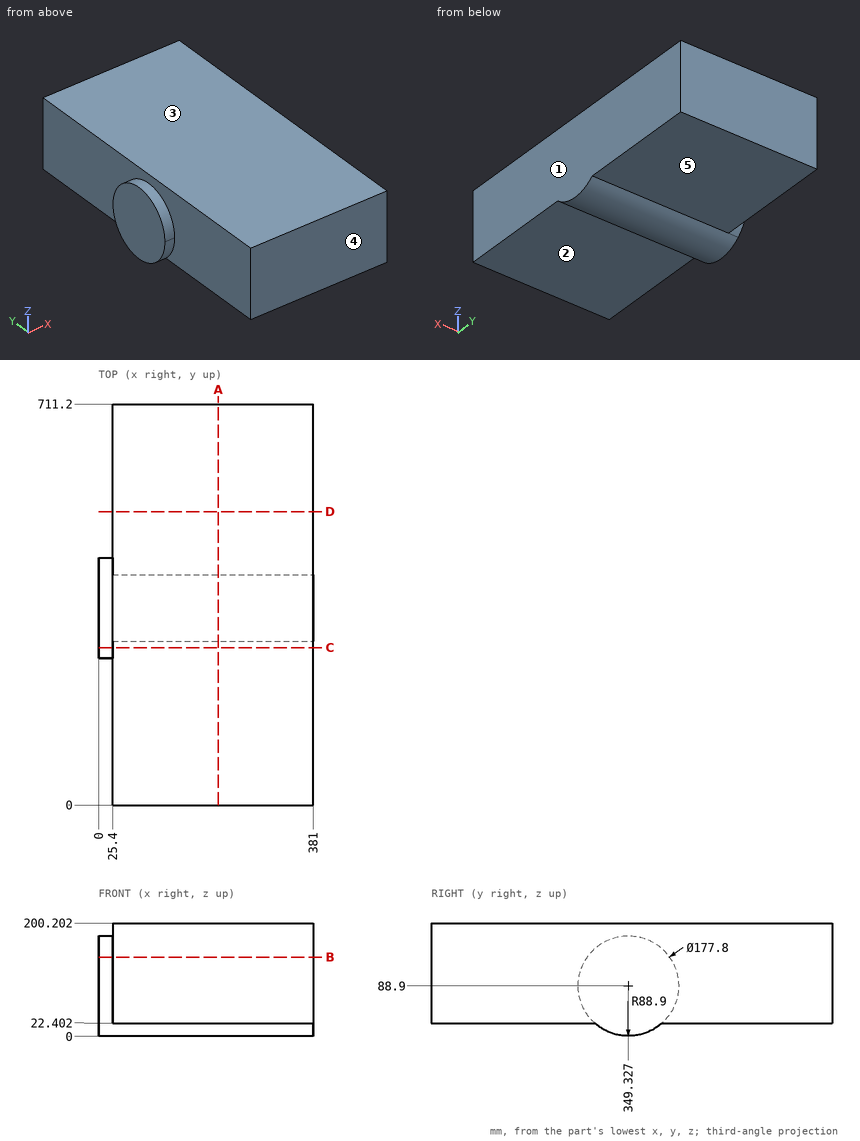
Input: dimensioned drawing with shaded views. Units: mm. Origin: part minimum x, y, z. A direction names the side the tool comes from. Coordinates: 2 decimals unless noted, no trailing zeros. Loops run counter-clockwise (first coordinate to the right, second up) from the corner with the lowest first, then second, coordinate; pieces in that order, holes last. Notation, with made-up numbers: (-7.75, 81) -> (44.25, 81) arc R23 ccw to (44.25, 96) -> close; hole circle Ø2 at (50, 80.5). An arc over 180 degrees is marked (long way). One line per item, written item: value. Start each with the question number.
Q1. Section query C-C, the plane y = 279. Return the cut outline in (x, z).
Q2. Mould query, pull axis Z, two halves, no side actions, for the marked faces 1, 2 and 3. Classes: pulls with the +Z half, pulls with the -Z half, needs draft (parallel to the pull), parting line crosses it, or undercut.
Q3. Contact query for flat-ended pins moving along their axis: P1, Ø1.5, axis at x = 52, y = 216, coming from the -Z side; P2, Ø1, axis at y = 474, z = 24, coming from the -X side. Output: stop coordinate, or through.
Q4. Section query B-B, the plane z = 140. Return the cut outline in (x, y).
Q5. Line query: line 1 along X through (y, z) = (533, 95); line 2 along Z through (x, y) = (41.5, 122); line 3 along Y through (x, z) = (108, 20). Output: solid intervals per line, ascending.
Q6. Section query A-A, the plane x = 212.5. Return the cut outline in (y, z).
Q7. Section query D-D, the plane y = 520.5. Return the cut outline in (x, z), and give its area (3 significant figures).
Q8. Set-up query: the marked faces 4 and 5. Return all of +Z, -Z, +X, -X, +Y, -Y with unobstructed straight access to the full face (end or side cutting, diameter ignored); none if empty.
Results:
1. outline: (0, 34.52) -> (25.4, 34.52) -> (25.4, 22.4) -> (381, 22.4) -> (381, 200.2) -> (25.4, 200.2) -> (25.4, 143.28) -> (0, 143.28) -> close
2. face 1: needs draft
2. face 2: pulls with the -Z half
2. face 3: pulls with the +Z half
3. P1: z = 22.4
3. P2: x = 25.4
4. outline: (0, 276.58) -> (25.4, 276.58) -> (25.4, 0) -> (381, 0) -> (381, 711.2) -> (25.4, 711.2) -> (25.4, 422.07) -> (0, 422.07) -> close
5. line 1: 25.4 to 381
5. line 2: 22.4 to 200.2
5. line 3: 293.15 to 405.51
6. outline: (0, 22.4) -> (290.33, 22.4) arc R88.9 ccw to (408.33, 22.4) -> (711.2, 22.4) -> (711.2, 200.2) -> (0, 200.2) -> close
7. outline: (25.4, 22.4) -> (381, 22.4) -> (381, 200.2) -> (25.4, 200.2) -> close
7. area: 63,200 mm^2
8. face 4: +Z, -Z, +X, -X, -Y
8. face 5: -Z, +X, -X, +Y
